The listing builds one solid part. Answer for the finished solid, in the listing's coordinates (mm). A direction names the side the tool comes from. Coordinates: 2 decimals unless noted, no trailing zeros. Order: outer loops, then holes, each group sorted by start corner. A loop starts at its lowest first (then second) coordinate and runs counter-clockwise, first axis right, second up. Notation, with made-up numbers: (72, -9.5) - (120, -9.5) arc R14 ccw to (120, 17.5) - close; hole circle Ø10 at (14.25, -34). An arc over 180 degrees is marked (long way). Use a Markdown table: item, result. Add a question column.
Item 1: Find the intervals of material crossed by line 1 along Z through (x, y) = (0, 5.75); line 2 along X through (y, z) = (103.5, -0.5); line 3 along Y through (x, z) = (-1.75, 1.75), in increasing order.
Item 2: The mould has two halves that part along Z. Classify faces 1 (the conical face through (-0.094, 157.759, 0.424)), 2 (the cylindrical face through (-1.08, 86.28, 4.88)), 3 (the flat face through (2, 0, 2)): released by +Z, released by -Z, zero draft, split by the parting line, or undercut.
Item 3: Flat-ended cylindrical pins translate along their axes: P1, Ø4, axis at y = 94.5, z = 1, coming from the +X side; P2, Ø1.5, axis at y = 87, z = -3, coming from the +X side; P3, Ø3, axis at x = -2.5, y = 84, coming from the -Z side; P4, Ø1.5, axis at x = -4, y = 67, coming from the +Z side. Find the tip coordinate at first contact, or state that the pin passes through.
Item 4: For faces 4 (the cylindrical face through (0.54, 166.89, 2.44)), 5 (the flat face through (2, 175, 2)), 6 (the cylindrical face through (-0.54, 8.11, 2.44)), determine the directions among +Z, -Z, +X, -X, +Y, -Y from which every point of the face is accessible in a straight line to the end or side of a thin tool.
Item 5: The part is cut by section A-A, the plane y = 90.5. Give the vertices of the cut face in (x, z).
from build123d import *

# Parameters (mm, degrees)
SKETCH2_R             = 5
BOSS_EXTRUDE2_DEPTH   = 175
M6_TAPPED_HOLE1_D     = 5
M6_TAPPED_HOLE1_DEPTH = 16
M6_TAPPED_HOLE1_TIP   = 1.502151548
M6_TAPPED_HOLE2_D     = 5
M6_TAPPED_HOLE2_DEPTH = 16
M6_TAPPED_HOLE2_TIP   = 1.502151548


with BuildPart() as part:
    # Sketch2 → Boss-Extrude2 (new body)
    with BuildSketch(Plane(origin=(0, 0, 0), x_dir=(1, 0, 0), z_dir=(0, 1, 0))):
        Circle(SKETCH2_R)
    extrude(amount=BOSS_EXTRUDE2_DEPTH)

    # M6 Tapped Hole1
    with Locations(Plane(origin=(0, 175, 0), x_dir=(1, 0, 0), z_dir=(0, 1, 0))):
        with Locations((0, 0)):
            Hole(M6_TAPPED_HOLE1_D / 2, depth=M6_TAPPED_HOLE1_DEPTH)
            with Locations((0, 0, -(M6_TAPPED_HOLE1_DEPTH + M6_TAPPED_HOLE1_TIP / 2))):  # 118° drill point
                Cone(0, M6_TAPPED_HOLE1_D / 2, M6_TAPPED_HOLE1_TIP, mode=Mode.SUBTRACT)

    # M6 Tapped Hole2
    with Locations(Plane(origin=(0, 0, 0), x_dir=(-1, 0, 0), z_dir=(0, -1, 0))):
        with Locations((0, 0)):
            Hole(M6_TAPPED_HOLE2_D / 2, depth=M6_TAPPED_HOLE2_DEPTH)
            with Locations((0, 0, -(M6_TAPPED_HOLE2_DEPTH + M6_TAPPED_HOLE2_TIP / 2))):  # 118° drill point
                Cone(0, M6_TAPPED_HOLE2_D / 2, M6_TAPPED_HOLE2_TIP, mode=Mode.SUBTRACT)


solid = part.part
Solution:
| question | item | result |
|---|---|---|
| 1 | line 1 | z = -5 to -2.5, 2.5 to 5 |
| 1 | line 2 | x = -4.97 to 4.97 |
| 1 | line 3 | y = 16.02 to 158.98 |
| 2 | face 1 | undercut |
| 2 | face 2 | split by the parting line |
| 2 | face 3 | zero draft |
| 3 | P1 | stops at x = 5 |
| 3 | P2 | stops at x = 4.47 |
| 3 | P3 | stops at z = -4.9 |
| 3 | P4 | stops at z = 3.8 |
| 4 | face 4 | +Y |
| 4 | face 5 | +Z, -Z, +X, -X, +Y |
| 4 | face 6 | -Y |
| 5 | outline | circle Ø10 at (0, 0) |
